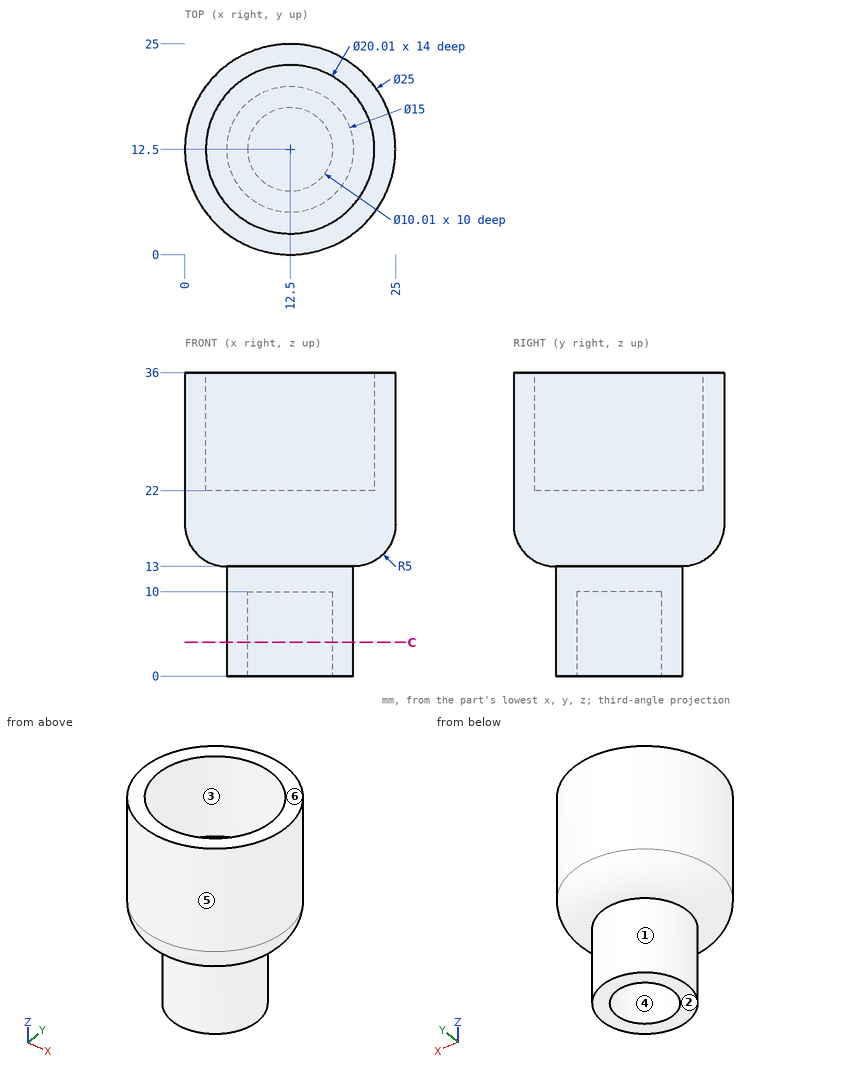
Can you work these out from the drawing? Everything is in mm from the part's minimum corner. A direction names the side the tool comes from. Give positions to 0.01 mm unless a question says otherwise; leave off trailing zeros. Write each loop counter-clockwise with the first axis right and the second up, starting at its lowest first coordinate (ties: lowest second). Pieces come first, ordered by that corner, then holes. Notation, with made-up numbers: M 84.5,-16 L 103.5,-16 A21 ccw 103.5,-8 Z; hole C -32.75,14.5 d4. An arc over 180 degrees is marked long. Answer in a Markdown table with one row per item. Add a question column.
Item 1: Imagine slicing it at C-C, the plane z = 4. Write out the boundary of the cut face in (x, y) (3 decimals), plus the area to 3 significant figures.
Item 2: Please list where these lines run through material, in increasing order: L1, parallel to Y at x = 12.5, z = 28.5 (3 decimals); L2, parallel to X at y = 15.75, z = 5.5; L3, parallel to Y at x = 12, z = 7.
Item 3: For pin 1 Ø2 at (x, z) = (9, 21.5) entering from +Y; pin 2 Ø7.5 at (x, y) = (12, 12) entering from -Z; pin 3 Ø3 at (x, y) = (17.5, 16.5) entering from +Z; pin 4 Ø8 at (x, z) = (13.5, 25) entering from +Y, each with a flat end and sliding along its axis, tell me the tip position at first contact or that it passes through.
Item 4: We'd pull the mould along Y, two halves only. Please class the marked faces 3, 4, 5 and 6: released by +Y, released by -Y, zero draft, split by the parting line, or undercut.
Item 5: On a 3-axis mill with a long thin cutter (end or side, diameter ignored), from which of +Z, -Z, +X, -X, +Y, -Y can I reach the whole of each face in a straight line? I mean the marked faces 1 and 2. Say none if no direction works.
Evaluation:
| question | item | result |
|---|---|---|
| 1 | outline | C 12.5,12.5 d15; hole C 12.5,12.5 d10.01 |
| 1 | area | 98.0 mm² |
| 2 | L1 | y = 0 to 2.495, 22.505 to 25 |
| 2 | L2 | x = 5.74 to 8.69, 16.31 to 19.26 |
| 2 | L3 | y = 5.02 to 7.52, 17.48 to 19.98 |
| 3 | pin 1 | stops at y = 24.75 |
| 3 | pin 2 | stops at z = 10 |
| 3 | pin 3 | stops at z = 22 |
| 3 | pin 4 | stops at y = 25 |
| 4 | face 3 | undercut |
| 4 | face 4 | undercut |
| 4 | face 5 | split by the parting line |
| 4 | face 6 | zero draft |
| 5 | face 1 | -Z |
| 5 | face 2 | -Z, +X, -X, +Y, -Y |
